Autodesk Inventor part; units mm, degrees
ref_plane "YZ Plane" through (0, 0, 0) normal (1, 0, 0) x (0, 1, 0)
ref_plane "XZ Plane" through (0, 0, 0) normal (0, 1, 0) x (-1, 0, 0)
ref_plane "XY Plane" through (0, 0, 0) normal (0, 0, 1) x (1, 0, 0)
sketch "Skizze1" plane through (0, 0, 0) normal (0, 0, 1) x (1, 0, 0)
  line L0 (0, -19.95) -> (0, 19.95) construction
  arc A0 (-5.5, -19.95) -> (5.5, -19.95) centre (0, -19.95) ccw
  arc A1 (5.5, 19.95) -> (-5.5, 19.95) centre (0, 19.95) ccw
  line L1 (0, 37.03) -> (0, -37.03) construction
  line L2 (-16.45, 0) -> (16.45, 0) construction
  circle A2 centre (0, 19.95) radius 1.5
  circle A3 centre (0, -19.95) radius 1.5
  circle A4 centre (0, 19.95) radius 6.5 construction
  circle A5 centre (0, -19.95) radius 6.5 construction
  line L3 (0, 26.45) -> (0, -26.45) construction
  circle A6 centre (0, 19.95) radius 2.5
  circle A7 centre (0, -19.95) radius 2.5
  circle A8 centre (0, 0) radius 9.75
  line L4 (-5.5, 19.95) -> (-5.5, 10.3833)
  line L5 (-5.5, -10.3833) -> (-5.5, -19.95)
  line L6 (5.5, -19.95) -> (5.5, -10.3833)
  line L7 (5.5, 10.3833) -> (5.5, 19.95)
  arc A9 (5.5, -10.3833) -> (5.5, 10.3833) centre (0, 0) ccw
  arc A10 (-5.5, 10.3833) -> (-5.5, -10.3833) centre (0, 0) ccw
  circle A11 centre (0, 0) radius 6.35 construction
  circle A12 centre (-4.4901, 4.4901) radius 1.5
  circle A13 centre (-4.4901, -4.4901) radius 1.5
  circle A14 centre (4.4901, -4.4901) radius 1.5
  circle A15 centre (4.4901, 4.4901) radius 1.5
  line L8 (-4.4901, 4.4901) -> (0, 0) construction
  dimension "d4" = 13
  dimension "d31" = 12.7
  dimension "d1" = 3
  dimension "d5" = 52.9
  dimension "d19" = 1
  dimension "d26" = 19.5
  dimension "d28" = 2
  dimension "d32" = 3
  dimension "d35" = 360
  dimension "d37" = 45
  dimension "d38" = 3
extrude "Extrusion1" add sketch "Skizze1" against normal blind 7 contours L5 A10 L4 A1 L7 A9 L6 A0 | A6 | A7
chamfer "Fase2" distance 2 distance2 7 6 edges at (5.5, -15.1666, 0) (0, -25.45, 0) (-5.5, -15.1666, 0) (0, 25.45, 0) (5.5, 15.1666, 0) (-5.5, 15.1666, 0) measured on face at (-4.0409, -16.4295, 0)
extrude "Extrusion4" add sketch "Skizze1" against normal blind 0.5 from surface at -7 contours A6 | A7
extrude "Extrusion6" add sketch "Skizze1" along normal blind 2 from surface at -7 contours A8
properties part number "HarmonicDrive-WaveGenerator-Bottom"
Input: part model. Units: mm. Frame: model coordinates. A direction names the side the tool comes from. Coordinates: 2 decimals unless noted, no trailing zeros. Loops run counter-clockwise (first coordinate to the right, second up) from the corner with the lowest first, then second, coordinate; pieces in that order, holes last. Notation, with made-up numbers: M -24.5,-11.75 L 4.5,-11.75 A24 cw 4.5,10.25 Z; hole C 80.25,37.5 d3. An arc over 180 degrees is marked long. Use a Markdown table: item, result. Add a question column.
1) Pin query (flat end, axial travel): P1, Ø4, axis at x = -7.5, z = -1.5, coming from the -Y side; P2, Ø1.8, axis at x = 4.49, y = 4.49, coming from the -Z side; P3, Ø8, axis at x = -2.5, y = 2, coming from the -Z side; P4, Ø1.5, axis at y = -10, z = -1.5, coming from the -X side. Return the tip coordinate at first contact, or that it passes through.
2) Section B-B, the plane y = 0. Return the cut outline in (x, z), plus the area to 3 significant figures.
3) Line query: L1, parallel to Y at x = -5.5, z = -6.25; L2, parallel to Y at x = -3.25, z = -6; L3, parallel to Y at x = -1, z = -1.25. Output: solid intervals per line, ascending. Write a range as from..to.
4) Section C-C, the plane z = -6.5. Return the cut outline in (x, y).
5) Draft query along Y for faces 1 (the flat face through (-4.5, 15.1, -3.5)), 2 (the cylindrical face through (-0.325, -21.414, -3.698)), 3 (the cylindrical face through (11.75, -0.21, -3.45)), 4 (the cylindrical face through (-5.68, -3.58, -6.01)). Return one class per face: +Y half, -Y half, draft (parallel to the pull), parting line (faces both ways), or undercut.
6) Section A-A, the plane x = 0. Give the number of separate pieces and of enclosed holes in the cut face, plus the area to 3 significant figures.
7) Set-up query: faces 5 (the cylindrical face through (-11.75, 0.21, -3.45)), 6 (the flat face through (4.5, -15.1, -3.5)), 7 (the flat face through (0, 0, -5)). Return all of +Z, -Z, +X, -X, +Y, -Y with unobstructed straight access to the full face (end or side cutting, diameter ignored); none if empty.
Answer below:
| question | item | result |
|---|---|---|
| 1 | P1 | y = -10.38 |
| 1 | P2 | through |
| 1 | P3 | z = -7 |
| 1 | P4 | x = -7.25 |
| 2 | outline | M -11.75,-7 L 11.75,-7 L 11.75,0 L 9.75,0 L 9.75,-5 L -9.75,-5 L -9.75,0 L -11.75,0 Z |
| 2 | area | 67.0 mm2 |
| 3 | L1 | -10.38..-5.6, -3.38..3.38, 5.6..10.38 |
| 3 | L2 | -24.03..-5.33, -3.65..3.65, 5.33..24.03 |
| 3 | L3 | -23.68..-21.07, -18.83..-9.7, 9.7..18.83, 21.07..23.68 |
| 4 | outline | M -5.36,-19.95 A5.36 ccw 5.36,-19.95 L 5.36,-10.46 A11.75 ccw 5.36,10.46 L 5.36,19.95 A5.36 ccw -5.36,19.95 L -5.36,10.46 A11.75 ccw -5.36,-10.46 Z; hole C -4.49,-4.49 d3; hole C -4.49,4.49 d3; hole C 0,-19.95 d3; hole C 0,19.95 d3; hole C 4.49,-4.49 d3; hole C 4.49,4.49 d3 |
| 5 | face 1 | draft |
| 5 | face 2 | undercut |
| 5 | face 3 | parting line |
| 5 | face 4 | undercut |
| 6 | separate pieces | 3 |
| 6 | enclosed holes | 0 |
| 6 | area | 205 mm2 |
| 7 | face 5 | +Z, -X |
| 7 | face 6 | +Z, +X, -Y |
| 7 | face 7 | +Z |
